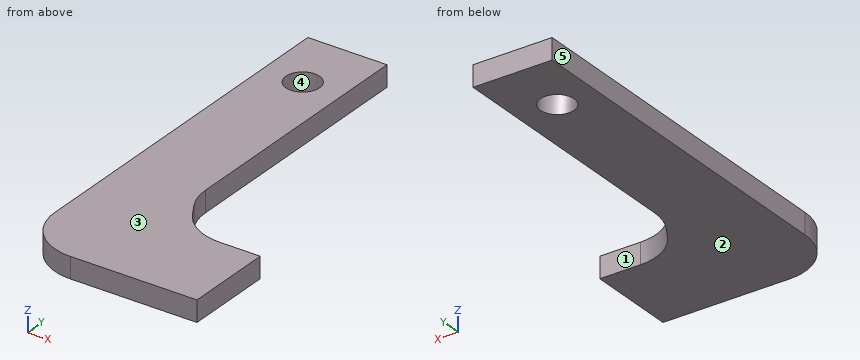
```python
from build123d import *

# Parameters (mm, degrees)
SKETCH_1_R      = 1.6
EXTRUDE_2_DEPTH = 2


with BuildPart() as part:
    # 草图1 → 凸台-拉伸2 (new body)
    with BuildSketch(Plane.XY):
        with BuildLine():
            Line((-13.587712402, 1.954995905), (-14.241535279, 3.056996382))
            ThreePointArc((-14.241535279, 3.056996382), (-14.763277187, 4.285507454), (-14.941422594, 5.608276628))
            Line((-14.941422594, 5.608276628), (-14.941422594, 30.006276151))
            Line((-14.941422594, 30.006276151), (-22.441422594, 30.006276151))
            Line((-22.441422594, 30.006276151), (-22.441422594, -3.993723849))
            ThreePointArc((-22.441422594, -3.993723849), (-20.9769565, -7.529257755), (-17.441422594, -8.993723849))
            Line((-17.441422594, -8.993723849), (-5.441422594, -8.993723849))
            Line((-5.441422594, -8.993723849), (-5.441422594, -0.493723849))
            Line((-5.441422594, -0.493723849), (-9.287599717, -0.493723849))
            ThreePointArc((-9.287599717, -0.493723849), (-11.761826745, 0.161371018), (-13.587712402, 1.954995905))
        make_face()
        with Locations((-18.691422594, 24.006276151)):
            Circle(SKETCH_1_R, mode=Mode.SUBTRACT)
    extrude(amount=EXTRUDE_2_DEPTH)


solid = part.part
```
Geometry check sheet. Reference: the model listing, model coordinates, mm. Face numbers are marked on the shaded views. A direction names the side the tool comes from. Coordinates: 2 decimals unless noted, no trailing zeros. Write each loop counter-clockwise with the first axis right and the second up, starting at its lowest first coordinate (ties: lowest second). Pieces come first, ordered by that corner, then holes. Notation, with made-up numbers: M 38,44.25 L 55,44.25 A6 cw 55,52.25 Z; hole C 42,-37.5 d1. An arc over 180 degrees is marked long. Use one line per item in the form item = value. Start each with the question number.
1) Section check A-A on z = 0.45. Enter the section's corners in (x, y) (3 decimals).
2) Section check C-C on x = -7.75. Enter the section's corners in (y, z), and give its area (3 significant figures).
3) Thickness scan on probe 1 along Y at (x, z) = (-7, 0.1); probe 2 along X at (y, z) = (22, 0.35); probe 3 along Y at (x, z) = (-18.5, 0.45). Record the ranges inside material, lowest first. Write a range as from..to.
4) Release check for a two-part mould opening along X. For the marked faces 3, 4 and 5 record: pulls with the +X half, pulls with the -X half, needs draft (parallel to the pull), parting line crosses it, or undercut.
5) Section check B-B on x = -19.5. Enter the section's corners in (y, z).
6) Set-up check for the marked faces 1 and 2: record each of +Z, -Z, +X, -X, +Y, -Y from which the full face is reachable in a straight line by a thin tool's end or side.
7) Section check D-D on y = 6.5. Enter the section's corners in (x, z), and give its area (3 significant figures).
Responses:
q1.outline = M -22.441,-3.994 A5 ccw -17.441,-8.994 L -5.441,-8.994 L -5.441,-0.494 L -9.288,-0.494 A5 cw -13.588,1.955 L -14.242,3.057 A5 cw -14.941,5.608 L -14.941,30.006 L -22.441,30.006 Z; hole C -18.691,24.006 d3.2
q2.outline = M -8.99,0 L -0.49,0 L -0.49,2 L -8.99,2 Z
q2.area = 17.0 mm2
q3.probe_1 = -8.99..-0.49
q3.probe_2 = -22.44..-14.94
q3.probe_3 = -8.88..22.42, 25.59..30.01
q4.face_3 = needs draft
q4.face_4 = undercut
q4.face_5 = pulls with the -X half
q5.outline = M -8.55,0 L 22.63,0 L 22.63,2 L -8.55,2 Z; M 25.39,0 L 30.01,0 L 30.01,2 L 25.39,2 Z
q6.face_1 = +Z, -Z, +X, +Y
q6.face_2 = -Z, +X, -X, +Y, -Y
q7.outline = M -22.44,0 L -14.94,0 L -14.94,2 L -22.44,2 Z
q7.area = 15.0 mm2
